from build123d import *

# Parameters (mm, degrees)
KUGGLUCKA_DEPTH     = 15
CIRPATTERN_COUNT    = 12
SKETCH1_R           = 1.754
CUT_EXTRUDE1_DEPTH  = 10
BOSS_EXTRUDE1_DEPTH = 10


with BuildPart() as part:
    # Ritning 1 → Kugghjulsämne (revolve)
    with BuildSketch(Plane.XY, mode=Mode.PRIVATE) as kugghjuls_mne_sk:
        Polygon((12.5, 1), (2.5, 1), (2.5, 3.5), (-12.5, 3.5), (-12.5, -3.5), (12.5, -3.5), align=None)
    revolve(kugghjuls_mne_sk.sketch.rotate(Axis((-12.5, -3.5, 0), (1, 0, 0)), 90), axis=Axis((-12.5, -3.5, 0), (1, 0, 0)))

    # Ritning 2 → Kugglucka (cut)
    with BuildSketch(Plane.ZY.offset(12.5)):
        with BuildLine():
            Line((1.419865071, 3.354486354), (0, 4.774351425))
            Line((0, 4.774351425), (-1.419865071, 3.354486354))
            add(Edge.make_bspline(
                [(-1.419865071, 3.354486354), (-1.173032372, 3.067088657), (-0.658113481, 2.467546927), (-0.604624671, 1.6768746), (-0.576776379, 1.265220772)],
                knots=[0, 0, 0, 0, 0.479362292, 1, 1, 1, 1], degree=3))
            ThreePointArc((-0.576776379, 1.265220772), (0, 1.3), (0.576776379, 1.265220772))
            add(Edge.make_bspline(
                [(1.419865071, 3.354486354), (1.173032372, 3.067088657), (0.658113481, 2.467546927), (0.604624671, 1.6768746), (0.576776379, 1.265220772)],
                knots=[0, 0, 0, 0, 0.479362292, 1, 1, 1, 1], degree=3))
        make_face()
    kugglucka = extrude(amount=-KUGGLUCKA_DEPTH, mode=Mode.SUBTRACT)

    # CirPattern: Kugglucka ×12 about axis
    cirpattern_axis = Axis((-12.5, -3.5, 0), (-1, 0, 0))
    for i in range(1, CIRPATTERN_COUNT):
        add(kugglucka.rotate(cirpattern_axis, i * 360 / CIRPATTERN_COUNT), mode=Mode.SUBTRACT)

    # Sketch1 → Cut-Extrude1 (cut)
    with BuildSketch(Plane(origin=(12.5, 0, 0), x_dir=(0, 0, -1), z_dir=(1, 0, 0))):
        with Locations((0, -3.5)):
            Circle(SKETCH1_R)
    extrude(amount=-CUT_EXTRUDE1_DEPTH, mode=Mode.SUBTRACT)

    # Sketch3 → Boss-Extrude1 (add)
    with BuildSketch(Plane(origin=(12.5, 0, 0), x_dir=(0, 0, -1), z_dir=(1, 0, 0))):
        Polygon((-1, -1.322696024), (-1, -6.208852365), (-3.330635242, -3.367112903), align=None)
    extrude(amount=-BOSS_EXTRUDE1_DEPTH)


solid = part.part
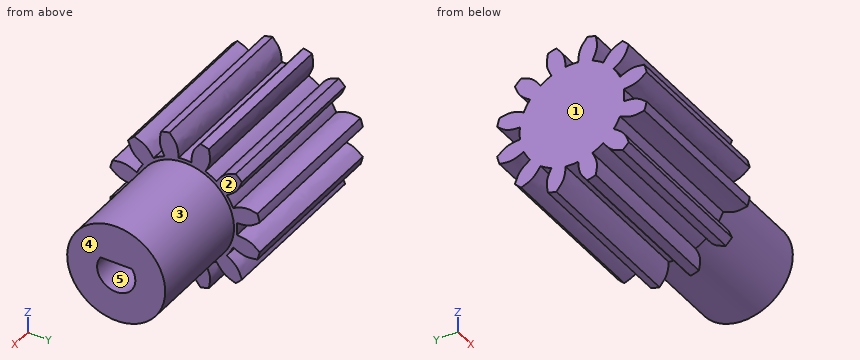
Geometry check sheet. Reference: the model listing, model coordinates, mm. Face numbers are marked on the shaded views. A direction names the side the tool comes from. Give positions to 0.01 mm unless a question says otherwise; leave off trailing zeros. Write each loop counter-clockwise with the first axis right and the second up, starting at its lowest first coordinate (ties: lowest second). Pieces come first, ordered by that corner, then holes. Notation, with made-up numbers: M -32,36.5 L 17,36.5 A19 ccw 17,40.5 Z; hole C -13.75,57 d3. An arc over 180 degrees is marked long. Answer as CSV lines item,"result". Start each with the question number.
Q1. Section check C-C, the plane y = -3.5. Record the cut outline in (x, z).
Q2. Go/stop test with flat-tipped pins: pin 1 (0.8 mm diameter, centred on y = -4, z = -0.5, fed in from +X); pin 2 (0.9 mm diameter, centred on x = 6, y = -4, fed in from -Z). Record where each tip stops, or that it passes through.
Q3. Release check for a two-part mould opening along Y. For the marked faces 3, 4 and 5 record: pulls with the +Y half, pulls with the -Y half, needs draft (parallel to the pull), parting line crosses it, or undercut.
Q4. Section check B-B, the plane x = 6. Record the cut outline in (y, z).
Q5. Material ranges on L1, parallel to Y at x = 8, z = 0; L2, parallel to Y at x = -3.5, z = -4.25; L3, parallel to Y at x = -11.5, z = -2, recorded low to high.
Q6. Tool access check on the marked faces 1 and 2. Record the directions out of +Z, -Z, +X, -X, +Y, -Y that give a thin tool (end or side, any length) a straight path to the whole face; none if there is none.
Q7. Section check A-A, the plane z = 0. Record the cut outline in (x, y).
Geometry says:
1,outline,"M -12.5,-4.8 L 2.5,-4.8 L 2.5,-4.5 L 12.5,-4.5 L 12.5,-1.75 L 2.5,-1.75 L 2.5,1 L 12.5,1 L 12.5,4.5 L 2.5,4.5 L 2.5,4.8 L -12.5,4.8 Z"
2,pin 1,"x = 2.5"
2,pin 2,"z = -4.5"
3,face 3,"parting line crosses it"
3,face 4,"needs draft"
3,face 5,"undercut"
4,outline,"C -3.5,0 d9; hole M -4.94,1 A1.75 ccw long -2.06,1 Z"
5,L1,"-8 to -5.25, -1.75 to 1"
5,L2,"-8.58 to -6.67, -5.73 to -1.27, -0.33 to 1.58"
5,L3,"-10.21 to -8.16, -7.86 to 0.86, 1.16 to 3.21"
6,face 1,"+Z, -Z, -X, +Y, -Y"
6,face 2,"+X"
7,outline,"M -12.5,-8.3 L 2.5,-8.3 L 2.5,-8 L 12.5,-8 L 12.5,-5.25 L 2.5,-5.25 L 2.5,-1.75 L 12.5,-1.75 L 12.5,1 L 2.5,1 L 2.5,1.3 L -12.5,1.3 Z"
